from build123d import *

# Parameters (mm, degrees)
SKETCH1_W           = 609.6
SKETCH1_H           = 609.6
BOSS_EXTRUDE1_DEPTH = 3.175
FILLET1_R           = 25.4
SKETCH2_W           = 12.7
SKETCH2_H           = 533.4
CUT_EXTRUDE1_DEPTH  = 3.175


with BuildPart() as part:
    # Sketch1 → Boss-Extrude1 (new body)
    with BuildSketch(Plane(origin=(0, 0, 0), x_dir=(1, 0, 0), z_dir=(0, 1, 0))):
        Rectangle(SKETCH1_W, SKETCH1_H)
    extrude(amount=BOSS_EXTRUDE1_DEPTH)

    # Fillet1
    fillet1_edges = [part.edges().sort_by_distance(p)[0] for p in [
        (304.8, 1.5875, 304.8),
        (-304.8, 1.5875, 304.8),
        (-304.8, 1.5875, -304.8),
        (304.8, 1.5875, -304.8),
    ]]
    fillet(fillet1_edges, radius=FILLET1_R)

    # Sketch2 → Cut-Extrude1 (cut)
    with BuildSketch(Plane(origin=(0, 3.175, 0), x_dir=(1, 0, 0), z_dir=(0, 1, 0))):
        with Locations((209.042, 0)):
            Rectangle(SKETCH2_W, SKETCH2_H)
        with Locations((-209.042, 0)):
            Rectangle(SKETCH2_W, SKETCH2_H)
        with Locations((-292.1, 0)):
            Rectangle(SKETCH2_W, SKETCH2_H)
        with Locations((292.1, 0)):
            Rectangle(SKETCH2_W, SKETCH2_H)
    extrude(amount=-CUT_EXTRUDE1_DEPTH, mode=Mode.SUBTRACT)


solid = part.part
Build history of the part. All positions in model axes, mm. Give positions to 0.01 mm unless a question says otherwise; leave off trailing zeros. Order: outer loops, then holes, each group sorted by start corner. A loop starts at its lowest first (then second) coordinate and runs counter-clockwise, first axis right, second up. Notation, with made-up numbers: M 17.5,5 L 36.5,5 A9 cw 36.5,15 Z; hole C 55.25,-20.75 d8. An arc over 180 degrees is marked long. Use one line per item in the form item = value.
Q1. Slice it at B-B, the plane y = 0.9. Write the cut outline in (x, z).
Conclusion:
outline = M -304.8,-279.4 A25.4 ccw -279.4,-304.8 L 279.4,-304.8 A25.4 ccw 304.8,-279.4 L 304.8,279.4 A25.4 ccw 279.4,304.8 L -279.4,304.8 A25.4 ccw -304.8,279.4 Z; hole M -298.45,-266.7 L -285.75,-266.7 L -285.75,266.7 L -298.45,266.7 Z; hole M -215.39,-266.7 L -202.69,-266.7 L -202.69,266.7 L -215.39,266.7 Z; hole M 202.69,-266.7 L 215.39,-266.7 L 215.39,266.7 L 202.69,266.7 Z; hole M 285.75,-266.7 L 298.45,-266.7 L 298.45,266.7 L 285.75,266.7 Z
Q2. Slice it at A-A, the plane z = 178.5. Write the cut outline in (x, y) (3 decimals), and give its area (3 significant figures).
Conclusion:
outline = M -304.8,0 L -298.45,0 L -298.45,3.175 L -304.8,3.175 Z; M -285.75,0 L -215.392,0 L -215.392,3.175 L -285.75,3.175 Z; M -202.692,0 L 202.692,0 L 202.692,3.175 L -202.692,3.175 Z; M 215.392,0 L 285.75,0 L 285.75,3.175 L 215.392,3.175 Z; M 298.45,0 L 304.8,0 L 304.8,3.175 L 298.45,3.175 Z
area = 1,770 mm2
Q3. Wall check: probe 1 along X at (y, z) = (0.45, -91); probe 2 along Z at (x, y) = (212.5, 1.2); probe 3 along X at (y, z) = (0.65, 280.5). Give the ranges that are in metal, low to high.
Conclusion:
probe_1 = -304.8 to -298.45, -285.75 to -215.39, -202.69 to 202.69, 215.39 to 285.75, 298.45 to 304.8
probe_2 = -304.8 to -266.7, 266.7 to 304.8
probe_3 = -304.78 to 304.78
Q4. Pin check, flat tips, straight feed: P1, Ø1, axis at x = -292, y = 2, coming from the +Z side; P2, Ø5, axis at x = -28.5, z = -92, coming from the -Y side. Stop position of each tip, or through.
Conclusion:
P1 = 301.73
P2 = 0
Q5. Pull direction X, two halves, no side cores. Call faces 1 (the cylindrical face through (297.56, 1.61, -297.16)), 2 (the cylindrical face through (-297.56, 1.61, -297.16)), 3 (the flat face through (-4, 3.175, -4)): released by +X, released by -X, zero draft, split by the parting line, or undercut.
Conclusion:
face_1 = released by +X
face_2 = released by -X
face_3 = zero draft
